```python
from build123d import *

# Parameters (mm, degrees)
F0_W     = 25.434012
F0_H     = 25.360106
F0_R     = 0.502726
F0_R_2   = 0.505177
F0_R_3   = 0.651682
F0_R_4   = 0.654036
F0_R_5   = 0.653901
F1_DEPTH = 5
F2_R     = 1
F3_R     = 1
F4_R     = 1
F5_R     = 1


with BuildPart() as f1:
    # F0 (on Top) → F1 (new body)
    with BuildSketch(Plane.XY):
        with Locations((-13.553905, -12.680053)):
            Rectangle(F0_W, F0_H)
        with Locations((-10.558297, -18.72582)):
            Circle(F0_R, mode=Mode.SUBTRACT)
        with Locations((-9.337448, -18.723993)):
            Circle(F0_R_2, mode=Mode.SUBTRACT)
        with Locations((-15.011093, -7.446084)):
            Circle(F0_R_3, mode=Mode.SUBTRACT)
        with Locations((-14.220849, -3.582401)):
            Circle(F0_R_4, mode=Mode.SUBTRACT)
        with Locations((-13.412111, -8.726368)):
            Circle(F0_R_5, mode=Mode.SUBTRACT)
    extrude(amount=F1_DEPTH)

    # F2
    f2_edges = [f1.edges().sort_by_distance(p)[0] for p in [
        (-13.553905, 0, 5),
    ]]
    fillet(f2_edges, radius=F2_R)

    # F3
    f3_edges = [f1.edges().sort_by_distance(p)[0] for p in [
        (-26.270911, -13.180053, 5),
    ]]
    fillet(f3_edges, radius=F3_R)

    # F4
    f4_edges = [f1.edges().sort_by_distance(p)[0] for p in [
        (-13.053905, -25.360106, 5),
    ]]
    fillet(f4_edges, radius=F4_R)

    # F5
    f5_edges = [f1.edges().sort_by_distance(p)[0] for p in [
        (-0.836899, -12.680053, 5),
    ]]
    fillet(f5_edges, radius=F5_R)


solid = f1.part
```
Check sheet for the modelled part. Datum: model origin and axes. Units: mm. Round coordinates to 2 decimals unless told otherwise and drop trailing zeros. Loops run counter-clockwise (first coordinate to the right, second up) from the corner with the lowest first, then second, coordinate; pieces in that order, holes last. Notation, with made-up numbers: (1.5, -8.75) - (56.5, -8.75) arc R3 cw to (56.5, -4.75) - close; hole circle Ø1 at (39.5, 85). An arc over 180 degrees is marked (long way). Write item = value, one per line. Start each with the question number.
Q1. Section check A-A (z = 4.7). Record the boundary of the cut face in (x, y), plus the area to 3 significant figures.
Q2. Release check for a two-part mould opening along X. For faces 1 (the face through (-10.667, -19.217, 2.465)), 2 (the face through (-14, -13, 0)), 3 (the face through (-1.12, -25.06, 2.03)), 4 (the face through (-13.931, -9.124, 2.465)) record: pulls with the +X half, pulls with the -X half, needs draft (parallel to the pull), parting line crosses it, or undercut.
Q3. Section check B-B (x = -9.25). Record the boundary of the cut face in (y, z), plus the area to 3 significant figures.
Q4. Thickness scan on L1, parallel to X at y = -19, z = 3.55; L2, parallel to Y at x = -9.75, z = 3.55; L3, parallel to Y at x = -15.5, z = 2.85. Record the ranges inside material, lowest first.
Q5. Depth check by flat-ended pin: P1, Ø0.9, axis at x = -9.34, y = -18.72, coming from the -Z side. Enter the tip coordinate at first touch or a pass-through.
Derived:
q1.outline = (-25.99, -24.36) arc R0.71 ccw to (-25.27, -25.07) - (-1.84, -25.07) arc R0.71 ccw to (-1.12, -24.36) - (-1.12, -1) arc R0.71 ccw to (-1.84, -0.29) - (-25.27, -0.29) arc R0.71 ccw to (-25.99, -1) - close; hole circle Ø1.3 at (-15.01, -7.45); hole circle Ø1.31 at (-14.22, -3.58); hole circle Ø1.31 at (-13.41, -8.73); hole circle Ø1.01 at (-10.56, -18.73); hole circle Ø1.01 at (-9.34, -18.72)
q1.area = 610 mm^2
q2.face_1 = undercut
q2.face_2 = needs draft
q2.face_3 = pulls with the +X half
q2.face_4 = undercut
q3.outline = (-25.36, 0) - (-19.22, 0) - (-19.22, 5) - (-24.36, 5) arc R1 ccw to (-25.36, 4) - close; (-18.23, 0) - (0, 0) - (0, 4) arc R1 ccw to (-1, 5) - (-18.23, 5) - close
q3.area = 121 mm^2
q4.L1 = -26.27 to -10.98, -10.14 to -9.76, -8.91 to -0.84
q4.L2 = -25.36 to -19.02, -18.43 to 0
q4.L3 = -25.36 to -7.88, -7.02 to 0
q5.P1 = through
